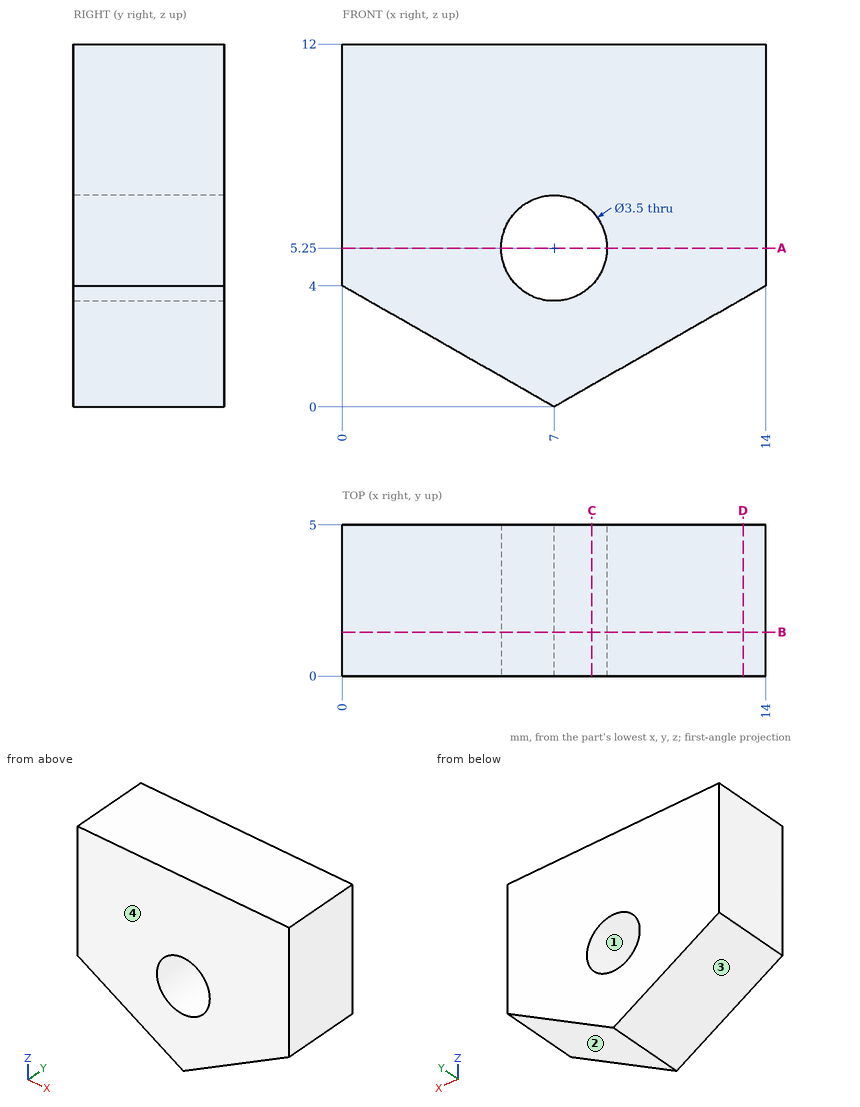
Geometry: see drawing. Coordinates: mm, zero at the bounding-box minimum. Round coordinates to 2 decimals unless told otherwise and drop trailing zeros. Order: outer loops, then holes, each group sorted by start corner. A loop starts at its lowest first (then second) coordinate and runs counter-clockwise, first axis right, second up. Notation, with made-up numbers: (-13, -29.75) - (-8, -29.75) arc R22 ccw to (-8, -3.75) - close; hole circle Ø4 at (16.5, 13). An arc over 180 degrees is marked (long way). Use a Markdown table: item, result. Add a question column.
1. Mould query, pull axis X, two halves, no side actions, for the marked faces 1, 2, 3 and 4. Classes: +X half, -X half, draft (parallel to the pull), parting line (faces both ways), or undercut.
2. Section query C-C (x = 8.25). Return the cut outline in (y, z).
3. Section query A-A (z = 5.25). Return the cut outline in (x, y).
4. Section query B-B (y = 1.45). Return the cut outline in (x, z).
5. Line query: probe 1 along X at (y, z) = (1.95, 5.25); probe 2 along X at (y, z) = (4.4, 6.5); probe 3 along Z at (x, y) = (7.5, 4.6). Output: solid intervals per line, ascending.
6. Section query D-D (x = 13.25). Return the cut outline in (y, z), then the cut area to 3 significant figures.
7. First-contact query: pin 1 (2 mm diameter, centred on x = 11, y = 3.5, fed in from -Z); pin 2 (1.5 mm diameter, centred on y = 3, z = 2, fed in from -X). Flat tips, straight axial feed; report the tip coordinate or a pass-through.
Derived:
| question | item | result |
|---|---|---|
| 1 | face 1 | undercut |
| 1 | face 2 | +X half |
| 1 | face 3 | -X half |
| 1 | face 4 | draft |
| 2 | outline | (0, 0.71) - (5, 0.71) - (5, 4.03) - (0, 4.03) - close; (0, 6.47) - (5, 6.47) - (5, 12) - (0, 12) - close |
| 3 | outline | (0, 0) - (5.25, 0) - (5.25, 5) - (0, 5) - close; (8.75, 0) - (14, 0) - (14, 5) - (8.75, 5) - close |
| 4 | outline | (0, 4) - (7, 0) - (14, 4) - (14, 12) - (0, 12) - close; hole circle Ø3.5 at (7, 5.25) |
| 5 | probe 1 | 0 to 5.25, 8.75 to 14 |
| 5 | probe 2 | 0 to 5.78, 8.22 to 14 |
| 5 | probe 3 | 0.29 to 3.57, 6.93 to 12 |
| 6 | outline | (0, 3.57) - (5, 3.57) - (5, 12) - (0, 12) - close |
| 6 | area | 42.1 mm2 |
| 7 | pin 1 | z = 1.71 |
| 7 | pin 2 | x = 2.19 |
